For this review, take the finished solid that the model builds, in its own axes (mm). A direction names the side the tool comes from. Give positions to 0.01 mm unless a question says otherwise; leave off trailing zeros. Write each loop counter-clockwise with the first axis right and the second up, starting at its lowest first coordinate (ties: lowest second). Pieces come first, ordered by that corner, then holes. Notation, with made-up numbers: (-4.75, 76.5) -> (12.25, 76.5) arc R17 ccw to (12.25, 109.5) -> close; hole circle Ø4 at (-7, 58). An arc over 180 degrees is marked (long way). Answer as CSV lines item,"result".
```python
from build123d import *

# Parameters (mm, degrees)
SKETCH_1_W          = 46.3
SKETCH_1_H          = 47
EXTRUDE_1_DEPTH     = 50
SKETCH_2_W          = 46.3
SKETCH_2_H          = 42
CUT_EXTRUDE_1_DEPTH = 32.3
SKETCH_3_W          = 42.3
SKETCH_3_H          = 40
CUT_EXTRUDE_2_DEPTH = 10
SKETCH_4_W          = 42.3
SKETCH_4_H          = 37
CUT_EXTRUDE_3_DEPTH = 8.7
SKETCH_5_W          = 2
SKETCH_5_H          = 22
SKETCH_5_W_2        = 26.3
SKETCH_5_H_2        = 2
CUT_EXTRUDE_4_DEPTH = 5
SKETCH_7_W          = 10
SKETCH_7_H          = 5
EXTRUDE_2_DEPTH     = 2
SKETCH_8_W          = 10
SKETCH_8_H          = 5
EXTRUDE_3_DEPTH     = 2
SKETCH_9_W          = 22
SKETCH_9_H          = 21.15
CUT_EXTRUDE_5_DEPTH = 6
SKETCH_11_R         = 2
EXTRUDE_4_DEPTH     = 4
SKETCH_12_R         = 2
CUT_EXTRUDE_6_DEPTH = 4
SCALE_1_SCALE       = 1.015


with BuildPart() as part:
    # 草圖1 → 填料-伸長1 (new body)
    with BuildSketch(Plane(origin=(0, 0, 0), x_dir=(1, 0, 0), z_dir=(0, 1, 0))):
        with Locations((23.15, 23.5)):
            Rectangle(SKETCH_1_W, SKETCH_1_H)
    extrude(amount=EXTRUDE_1_DEPTH)

    # 草圖2 → 除料-伸長1 (cut)
    with BuildSketch(Plane(origin=(0, 50, 0), x_dir=(1, 0, 0), z_dir=(0, 1, 0))):
        with Locations((23.15, 21)):
            Rectangle(SKETCH_2_W, SKETCH_2_H)
    extrude(amount=-CUT_EXTRUDE_1_DEPTH, mode=Mode.SUBTRACT)

    # 草圖3 → 除料-伸長2 (cut)
    with BuildSketch(Plane(origin=(0, 17.7, 0), x_dir=(1, 0, 0), z_dir=(0, 1, 0))):
        with Locations((23.15, 22)):
            Rectangle(SKETCH_3_W, SKETCH_3_H)
    extrude(amount=-CUT_EXTRUDE_2_DEPTH, mode=Mode.SUBTRACT)

    # 草圖4 → 除料-伸長3 (cut, through all)
    with BuildSketch(Plane(origin=(0, 7.7, 0), x_dir=(1, 0, 0), z_dir=(0, 1, 0))):
        with Locations((23.15, 23.5)):
            Rectangle(SKETCH_4_W, SKETCH_4_H)
    extrude(amount=-CUT_EXTRUDE_3_DEPTH, mode=Mode.SUBTRACT)

    # 草圖5 → 除料-伸長4 (cut)
    with BuildSketch(Plane(origin=(0, 17.7, 0), x_dir=(1, 0, 0), z_dir=(0, 1, 0))):
        with Locations((1, 21)):
            Rectangle(SKETCH_5_W, SKETCH_5_H)
        with Locations((45.3, 21)):
            Rectangle(SKETCH_5_W, SKETCH_5_H)
        with Locations((23.15, 1)):
            Rectangle(SKETCH_5_W_2, SKETCH_5_H_2)
    extrude(amount=-CUT_EXTRUDE_4_DEPTH, mode=Mode.SUBTRACT)

    # 草圖7 → 填料-伸長2 (add)
    with BuildSketch(Plane.ZY):
        with BuildLine():
            Line((-42, 32.7), (-42, 22.7))
            Line((-42, 22.7), (-32, 22.7))
            ThreePointArc((-32, 22.7), (-34.928932188, 29.771067812), (-42, 32.7))
        make_face()
        with Locations((-37, 20.2)):
            Rectangle(SKETCH_7_W, SKETCH_7_H)
    extrude(amount=-EXTRUDE_2_DEPTH)

    # 草圖8 → 填料-伸長3 (add)
    with BuildSketch(Plane(origin=(46.3, 0, 0), x_dir=(0, 0, -1), z_dir=(1, 0, 0))):
        with Locations((37, 20.2)):
            Rectangle(SKETCH_8_W, SKETCH_8_H)
        with BuildLine():
            Line((32, 22.7), (42, 22.7))
            Line((42, 22.7), (42, 32.7))
            ThreePointArc((42, 32.7), (34.928932188, 29.771067812), (32, 22.7))
        make_face()
    extrude(amount=-EXTRUDE_3_DEPTH)

    # 草圖9 → 除料-伸長5 (cut, through all)
    with BuildSketch(Plane.XY.offset(-42)):
        with BuildLine():
            ThreePointArc((34.15, 28.85), (23.15, 17.85), (12.15, 28.85))
            Line((12.15, 28.85), (34.15, 28.85))
        make_face()
        with Locations((23.15, 39.425)):
            Rectangle(SKETCH_9_W, SKETCH_9_H)
    extrude(amount=-CUT_EXTRUDE_5_DEPTH, mode=Mode.SUBTRACT)

    # 草圖11 → 填料-伸長4 (add)
    with BuildSketch(Plane.XZ):
        with BuildLine():
            Line((51.3, -5), (46.3, -5))
            Line((46.3, -5), (46.3, -15))
            Line((46.3, -15), (51.3, -15))
            ThreePointArc((51.3, -15), (56.3, -10), (51.3, -5))
        make_face()
        with Locations((51.3, -10)):
            Circle(SKETCH_11_R, mode=Mode.SUBTRACT)
        with BuildLine():
            Line((46.3, -32), (46.3, -42))
            Line((46.3, -42), (51.3, -42))
            ThreePointArc((51.3, -42), (56.3, -37), (51.3, -32))
            Line((51.3, -32), (46.3, -32))
        make_face()
        with Locations((51.3, -37)):
            Circle(SKETCH_11_R, mode=Mode.SUBTRACT)
        with BuildLine():
            Line((0, -15), (0, -5))
            Line((0, -5), (-5, -5))
            ThreePointArc((-5, -5), (-10, -10), (-5, -15))
            Line((-5, -15), (0, -15))
        make_face()
        with BuildLine():
            Line((0, -42), (0, -32))
            Line((0, -32), (-5, -32))
            ThreePointArc((-5, -32), (-10, -37), (-5, -42))
            Line((-5, -42), (0, -42))
        make_face()
        with Locations((-5, -37)):
            Circle(SKETCH_11_R, mode=Mode.SUBTRACT)
    extrude(amount=-EXTRUDE_4_DEPTH)

    # 草圖12 → 除料-伸長6 (cut)
    with BuildSketch(Plane.XZ):
        with Locations((-5, -10)):
            Circle(SKETCH_12_R)
    extrude(amount=-CUT_EXTRUDE_6_DEPTH, mode=Mode.SUBTRACT)


with BuildPart() as part_1:
    # 縮放比例1: scaled about (23.15, 15.034187995, -32.143313771)
    add(part.part.scale(SCALE_1_SCALE).moved(Location((-0.34725, -0.22551282, 0.482149707))))


solid = part_1.part
```
Q1. To check wall thickness, follow probe 1 along X at (y, z) = (21.5, -39); probe 2 along Z at (x, y) = (12.5, 9.5); probe 3 along X at (y, z) = (17.5, -1.5). State the ranges of each line that lie inside material, in increasing order. Write a range as [from, to].
Answer block:
probe 1,"x = [-0.35, 1.68], [44.62, 46.65]"
probe 2,"z = [-47.22, -42.15], [-1.55, 0.48]"
probe 3,"x = [-0.35, 9.8], [36.5, 46.65]"
Q2. Clearance check with flat-ended pins moving along their axes: pin 1 (11 mm diameter, centred on x = -5, z = -39, fed in from +Y); pin 2 (1.2 mm diameter, centred on x = 48.5, y = 1.5, fed in from +Z); pin 3 (4 mm diameter, centred on x = 38, z = -39, fed in from -Y); pin 4 (1 mm diameter, centred on x = 1, y = 19.5, fed in from +Z). State where each tip first meets the part, or that it passes through.
Answer block:
pin 1,"stops at y = 32.96"
pin 2,"stops at z = -4.59"
pin 3,"passes through"
pin 4,"stops at z = -32"
Q3. Add section B-B (x = 23.15). Write out the cut boundary in (y, z).
Answer block:
outline,"(-0.23, -47.22) -> (17.89, -47.22) -> (17.89, -42.15) -> (-0.23, -42.15) -> close; (-0.23, -4.59) -> (7.59, -4.59) -> (7.59, -1.55) -> (12.66, -1.55) -> (12.66, 0.48) -> (-0.23, 0.48) -> close"
Q4. Draft analysis for pull direction X (two halves, no side actions). For faces 4 (the flat face through (23, 7.59, -3)), 5 (the flat face through (46, 15, -9.668)), 6 (the cylindrical face through (-10.496, 1.776, -9.556)), state which applies: released by +X, released by -X, zero draft, split by the parting line, or undercut.
Answer block:
face 4,"undercut"
face 5,"zero draft"
face 6,"released by -X"
Q5. Add section D-D (y = 34). Write out the cut boundary in (x, z) (3 decimals).
Answer block:
outline,"(-0.347, -47.223) -> (11.985, -47.223) -> (11.985, -42.148) -> (-0.347, -42.148) -> close; (34.315, -47.223) -> (46.647, -47.223) -> (46.647, -42.148) -> (34.315, -42.148) -> close"
Q6. Add section A-A (y = 10.5). Write out the cut boundary in (x, z), plus the area to 3 significant figures.
Answer block:
outline,"(-0.35, -47.22) -> (46.65, -47.22) -> (46.65, 0.48) -> (-0.35, 0.48) -> close; hole (1.68, -42.15) -> (44.62, -42.15) -> (44.62, -1.55) -> (1.68, -1.55) -> close"
area,"499 mm2"
Q7. For faces 1 (the flat face through (23, 4, -4.593)), 2 (the flat face through (-3, 3.834, -10)), 3 (the flat face through (34.315, 40, -45)), list the 3-axis set-ups (+Z, -Z, +X, -X, +Y, -Y) from which the entire face can be reached by the end or side of a thin tool; tool diameter is ignored.
Answer block:
face 1,"+Y, -Y"
face 2,"+Z, -Z, -X, +Y"
face 3,"+Z, -Z, +Y"
Q8. Add section C-C (z = -5.5). Write out the cut boundary in (x, y), plus the area to 3 significant figures.
Answer block:
outline,"(-8.32, -0.23) -> (1.68, -0.23) -> (1.68, 17.74) -> (-0.35, 17.74) -> (-0.35, 3.83) -> (-8.32, 3.83) -> close; (44.62, -0.23) -> (54.62, -0.23) -> (54.62, 3.83) -> (46.65, 3.83) -> (46.65, 17.74) -> (44.62, 17.74) -> close"
area,"138 mm2"
